Build history of the part. All positions in model axes, mm. A direction names the side the tool comes from. Coordinates: 2 decimals unless noted, no trailing zeros. Loops run counter-clockwise (first coordinate to the right, second up) from the corner with the lowest first, then second, coordinate; pieces in that order, holes last.
Item 1: 3-axis set-ups, long thin cutter, end or side, ignore diameter. For faces 5 (the face through (3, -3, 20)), 6 (the face through (2, -6, 8)), 7 (the face through (-2.17, -9.76, -1.52)), 8 (the face through (0, -7, -3)), 9 (the face through (2, -6, 5)): which of +Z, -Z, +X, -X, +Y, -Y reach the whole face in a straight line?
Item 2: Cut at A-A (x = 6.5). List the corners of the cut face in (y, z).
Item 3: Mould opens along Y. For faces 1 (the face through (3, -3, -15)), 2 (the face through (-6, 0, 2)), 3 (the face through (0, 0, -5)), 4 (the face through (-2.539, -1.947, -9.93)) say: released by +Y, released by -Y, zero draft, split by the parting line, or undercut.
Item 4: Drill centre lines: line 1 along Y through (x, z) = (0, -10.75); line 2 along Z through (x, y) = (-4.5, -6.5); line 3 along Y through (x, z) = (-1.25, -11). Where is each one in solid material? Low to high.
Item 5: Flat gauge pins, fed straight in: pin 1 (10 mm diameter, centred on x = 3, z = 13.5, fed in from +Y); pin 2 (5 mm diameter, centred on x = 1.5, y = -0.5, fed in from -Z); pin 3 (8 mm diameter, centred on x = -6.5, z = 7.5, fed in from +Y); pin 4 (3 mm diameter, centred on x = 0, z = 2, fed in from -Y). Where does each tip first touch, or does it go through?
Item 6: Cut at B-B (y = 0). List the corners of the cut face in (x, z), and give its area (3 significant figures).
Item 7: Cut at D-D (z = 12). List the corners of the cut face in (x, y), and give its area (3 significant figures).
from build123d import *

# Parameters (mm, degrees)
REAR_FLANGE_START    = -3
SKETCH1_R            = 10
REAR_FLANGE_DEPTH    = 3
SKETCH2_R            = 6
THROUGH_BODY_DEPTH   = 5
LOCK_NUT_START       = 5
SKETCH3_R            = 9
LOCK_NUT_DEPTH       = 3
INSIDE_PORT_START    = 8
SKETCH4_R            = 6
INSIDE_PORT_DEPTH    = 12
INSIDE_SOCKET_START  = 20
SKETCH5_R            = 3.2
INSIDE_SOCKET_DEPTH  = 10
OUTSIDE_PORT_START   = -15
SKETCH6_R            = 6
OUTSIDE_PORT_DEPTH   = 12
OUTSIDE_SOCKET_START = -5
SKETCH7_R            = 3.2
OUTSIDE_SOCKET_DEPTH = 10


with BuildPart() as part:
    # Sketch1 → Rear_Flange (new body)
    with BuildSketch(Plane.XY.offset(REAR_FLANGE_START)):
        Circle(SKETCH1_R)
    extrude(amount=REAR_FLANGE_DEPTH)

    # Sketch2 → Through_Body (add)
    with BuildSketch(Plane.XY):
        Circle(SKETCH2_R)
    extrude(amount=THROUGH_BODY_DEPTH)

    # Sketch3 → Lock_Nut (add)
    with BuildSketch(Plane.XY.offset(LOCK_NUT_START)):
        Circle(SKETCH3_R)
    extrude(amount=LOCK_NUT_DEPTH)

    # Sketch4 → Inside_Port (add)
    with BuildSketch(Plane.XY.offset(INSIDE_PORT_START)):
        Circle(SKETCH4_R)
    extrude(amount=INSIDE_PORT_DEPTH)

    # Sketch5 → Inside_Socket (cut)
    with BuildSketch(Plane.XY.offset(INSIDE_SOCKET_START)):
        Circle(SKETCH5_R)
    extrude(amount=-INSIDE_SOCKET_DEPTH, mode=Mode.SUBTRACT)

    # Sketch6 → Outside_Port (add)
    with BuildSketch(Plane.XY.offset(OUTSIDE_PORT_START)):
        Circle(SKETCH6_R)
    extrude(amount=OUTSIDE_PORT_DEPTH)

    # Sketch7 → Outside_Socket (cut)
    with BuildSketch(Plane.XY.offset(OUTSIDE_SOCKET_START)):
        Circle(SKETCH7_R)
    extrude(amount=-OUTSIDE_SOCKET_DEPTH, mode=Mode.SUBTRACT)


solid = part.part
Filled sheet:
1. face 5: +Z, +X, -X, +Y, -Y
1. face 6: +Z
1. face 7: +Z, -Z
1. face 8: -Z
1. face 9: none
2. outline: (-7.6, -3) - (7.6, -3) - (7.6, 0) - (-7.6, 0) - close; (-6.22, 5) - (6.22, 5) - (6.22, 8) - (-6.22, 8) - close
3. face 1: zero draft
3. face 2: split by the parting line
3. face 3: undercut
3. face 4: undercut
4. line 1: y = -6 to -3.2, 3.2 to 6
4. line 2: z = -3 to 0, 5 to 8
4. line 3: y = -5.87 to -2.95, 2.95 to 5.87
5. pin 1: stops at y = 6
5. pin 2: stops at z = -15
5. pin 3: stops at y = 8.65
5. pin 4: stops at y = -6
6. outline: (-10, -3) - (-6, -3) - (-6, -15) - (-3.2, -15) - (-3.2, -5) - (3.2, -5) - (3.2, -15) - (6, -15) - (6, -3) - (10, -3) - (10, 0) - (6, 0) - (6, 5) - (9, 5) - (9, 8) - (6, 8) - (6, 20) - (3.2, 20) - (3.2, 10) - (-3.2, 10) - (-3.2, 20) - (-6, 20) - (-6, 8) - (-9, 8) - (-9, 5) - (-6, 5) - (-6, 0) - (-10, 0) - close
6. area: 334 mm2
7. outline: circle Ø12 at (0, 0); hole circle Ø6.4 at (0, 0)
7. area: 80.9 mm2
